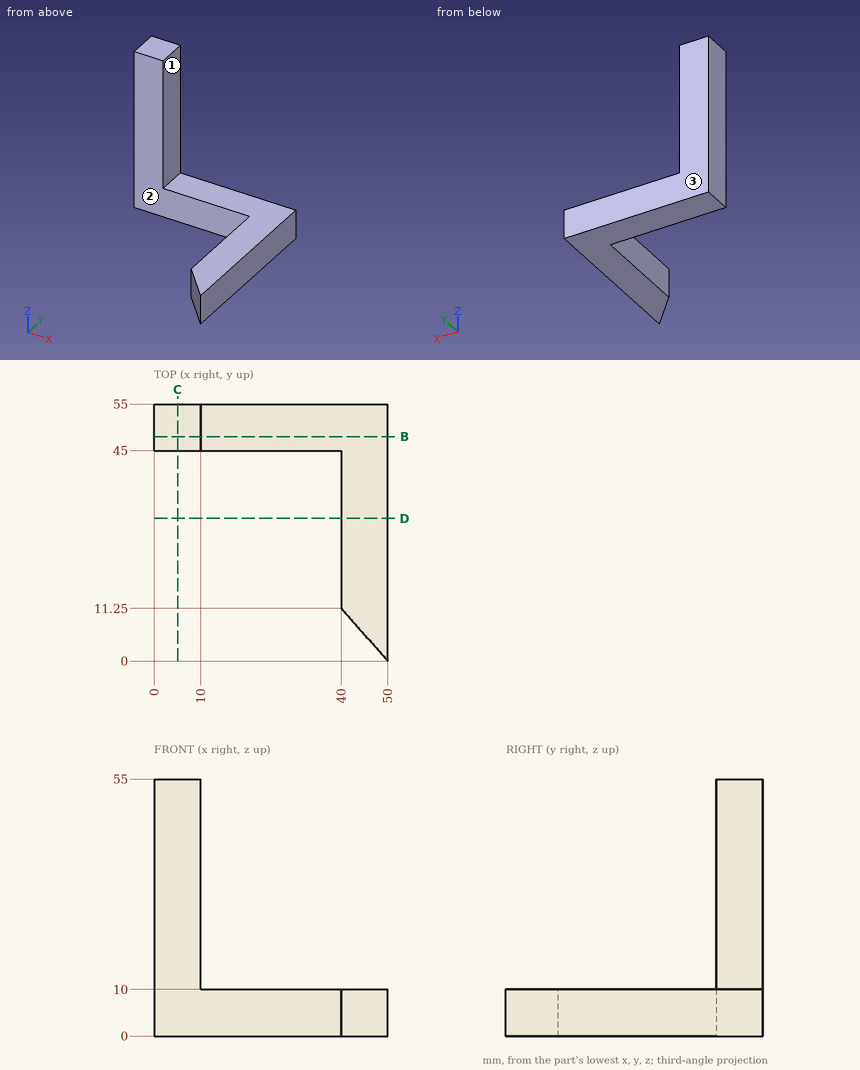
Can you work these out from the drawing? Everything is in mm from the part's minimum corner. A direction names the side the tool comes from. Round coordinates to 2 decimals unless told otherwise and drop trailing zeros. Loops run counter-clockwise (first coordinate to the right, second up) from the corner with the lowest first, then second, coordinate; pieces in that order, holes last. Notation, with made-up numbers: (35, -4) - (44, -4) arc R14 cw to (44, 22) - close; hole circle Ø11 at (34, 29.5). An arc over 180 degrees is marked (long way). Answer in a Markdown table with one row per item. Add a question column.
Q1. I want a section at B-B on y = 48. List the corners of the cut face in (x, z) for me.
Q2. For pin 1 Ø3 at (y, z) = (51.5, 30) entering from +X; pin 2 Ø5 at (y, z) = (33, 6) entering from -X; pin 3 Ø8 at (x, z) = (35.5, 12) entering from -Y, each with a flat end and sliding along its axis, tell me the tip position at first contact or that it passes through.
Q3. Which directions (+Z, -Z, +X, -X, +Y, -Y) give clear straight access to the entire face, cutting with the end or side of a thin tool? Please do the marked faces 1, 2 and 3.
Q4. I need wall thicknesses on L1, parallel to X at y = 47, z = 31.5; L2, parallel to Y at x = 3, z = 34. Which ranges of each line are inside material? Lowest first, please.
Q5. I want a section at C-C on x = 5. List the corners of the cut face in (y, z) for me, and give its area (3 significant figures).
Q6. I want a section at D-D on y = 30.5. List the corners of the cut face in (x, z) for me.
A:
| question | item | result |
|---|---|---|
| 1 | outline | (0, 0) - (50, 0) - (50, 10) - (10, 10) - (10, 55) - (0, 55) - close |
| 2 | pin 1 | x = 10 |
| 2 | pin 2 | x = 40 |
| 2 | pin 3 | y = 45 |
| 3 | face 1 | +Z, +X, +Y, -Y |
| 3 | face 2 | +Z, -Z, -X, -Y |
| 3 | face 3 | +Z, -Z, +X, -X, +Y |
| 4 | L1 | 0 to 10 |
| 4 | L2 | 45 to 55 |
| 5 | outline | (45, 0) - (55, 0) - (55, 55) - (45, 55) - close |
| 5 | area | 550 mm^2 |
| 6 | outline | (40, 0) - (50, 0) - (50, 10) - (40, 10) - close |
